from build123d import *

# Parameters (mm, degrees)
ESBO_O1_R                = 40
RESSALTO_EXTRUS_O1_DEPTH = 1
ESBO_O3_R                = 3.5
RESSALTO_EXTRUS_O2_DEPTH = 2
ESBO_O4_R                = 2.5
CORTE_EXTRUS_O2_DEPTH    = 2
CHANFRO1_SIZE            = 2
ESBO_O6_R                = 1.1
CORTE_EXTRUS_O4_DEPTH    = 3
CORTE_EXTRUS_O5_START    = -3
CORTE_EXTRUS_O5_DEPTH    = 3
ESBO_O7_W                = 38.307647293
ESBO_O7_H                = 77.740133008
CORTE_EXTRUS_O6_DEPTH    = 3
FILETE1_R                = 20
FILETE2_R                = 20


with BuildPart() as part:
    # Esboço1 → Ressalto-extrusão1 (new body)
    with BuildSketch(Plane(origin=(0, 0, 0), x_dir=(1, 0, 0), z_dir=(0, 1, 0))):
        with Locations(Location((0, 0, 0), (0, 0, 270))):
            Circle(ESBO_O1_R)
    extrude(amount=RESSALTO_EXTRUS_O1_DEPTH)

    # Esboço3 → Ressalto-extrusão2 (add)
    with BuildSketch(Plane(origin=(0, 1, 0), x_dir=(1, 0, 0), z_dir=(0, 1, 0))):
        with Locations(Location((0, 0, 0), (0, 0, 270))):
            Circle(ESBO_O3_R)
    extrude(amount=RESSALTO_EXTRUS_O2_DEPTH)

    # Esboço4 → Corte-extrusão2 (cut)
    with BuildSketch(Plane(origin=(0, 3, 0), x_dir=(1, 0, 0), z_dir=(0, 1, 0))):
        with Locations(Location((0, 0, 0), (0, 0, 270))):
            Circle(ESBO_O4_R)
    extrude(amount=-CORTE_EXTRUS_O2_DEPTH, mode=Mode.SUBTRACT)

    # Chanfro1
    chanfro1_edges = [part.edges().sort_by_distance(p)[0] for p in [
        (0, 1, -3.5),
    ]]
    chamfer(chanfro1_edges, length=CHANFRO1_SIZE - 0.0001)  # a hair under: the kernel refuses the full size

    # Esboço6 → Corte-extrusão4 (cut)
    with BuildSketch(Plane(origin=(0, 1, 0), x_dir=(1, 0, 0), z_dir=(0, 1, 0))):
        with Locations(Location((0, 0, 0), (0, 0, 270))):
            Circle(ESBO_O6_R)
    extrude(amount=-CORTE_EXTRUS_O4_DEPTH, mode=Mode.SUBTRACT)

    # Esboço2 → Corte-extrusão5 (cut)
    with BuildSketch(Plane(origin=(0, 1, 0), x_dir=(1, 0, 0), z_dir=(0, 1, 0)).offset(CORTE_EXTRUS_O5_START)):
        with BuildLine():
            ThreePointArc((20, 4), (16, 0), (20, -4))
            Line((20, -4), (39.223227028, -7.844645406))
            ThreePointArc((39.223227028, -7.844645406), (40, 0), (39.223227028, 7.844645406))
            Line((39.223227028, 7.844645406), (20, 4))
        make_face()
    extrude(amount=CORTE_EXTRUS_O5_DEPTH, mode=Mode.SUBTRACT)

    # Esboço7 → Corte-extrusão6 (cut)
    with BuildSketch(Plane(origin=(0, 1, 0), x_dir=(1, 0, 0), z_dir=(0, 1, 0))):
        with Locations((-28.594052983, 0)):
            Rectangle(ESBO_O7_W, ESBO_O7_H)
    extrude(amount=-CORTE_EXTRUS_O6_DEPTH, mode=Mode.SUBTRACT)

    # Filete1
    filete1_edges = [part.edges().sort_by_distance(p)[0] for p in [
        (-9.440229337, 0.5, -38.870066504),
    ]]
    fillet(filete1_edges, radius=FILETE1_R)

    # Filete2
    filete2_edges = [part.edges().sort_by_distance(p)[0] for p in [
        (-9.440229337, 0.5, 38.870066504),
    ]]
    fillet(filete2_edges, radius=FILETE2_R)


solid = part.part
Design review of the part built by this model. Coordinates are the model's own, in mm. A direction names the side the tool comes from. Coordinates: 2 decimals unless noted, no trailing zeros. Write each loop counter-clockwise with the first axis right and the second up, starting at its lowest first coordinate (ties: lowest second). Pieces come first, ordered by that corner, then holes. Notation, with made-up numbers: (39.5, -27) - (67.5, -27) arc R19 ccw to (67.5, -22) - close; hole circle Ø11 at (68.25, 27). An arc over 180 degrees is marked (long way). One line per item, written item: value.
1) For faces 1 (the face through (-2.44, 2.01, -0.54)), 2 (the face through (29.75, 0.49, -5.95)), 3 (the face through (1.09, 0.51, -0.14)), list the 3-axis set-ups (+Z, -Z, +X, -X, +Y, -Y) from which the entire face can be reached by the end or side of a thin tool; tool diameter is ignored.
Answer sheet:
face 1: +Y
face 2: +X, +Y, -Y
face 3: +Y, -Y
2) Add section D-D (z = -16). State the section outline as (x, y) points, plus the area to 3 significant figures.
Answer sheet:
outline: (-9.44, 0) - (36.66, 0) - (36.66, 1) - (-9.44, 1) - close
area: 46.1 mm2
3) Add section A-A (x = 24). State the section outline as (y, z) points.
Answer sheet:
outline: (0, -32) - (1, -32) - (1, -4.8) - (0, -4.8) - close; (0, 4.8) - (1, 4.8) - (1, 32) - (0, 32) - close
4) Insertion check: pin 1 (8 mm diameter, centred on x = 25.5, z = -3.5, fed in from -Y); pin 2 (1 mm diameter, centred on x = 11, z = 29, fed in from +Y); pin 3 (1.5 mm diameter, centred on x = 6, y = 1, fed in from +Z). Each pin has a flat end and moves straight along its axis. Give the tip position at first contact, or say it passes through.
Answer sheet:
pin 1: stops at y = 0
pin 2: stops at y = 1
pin 3: stops at z = 36.62
5) Mouldability with a two-part tool opening along X and no side actions: class faces 4 (the face through (-1, 1, 1)), 5 (the face through (33.01, 0.49, -22.59)), 6 (the face through (10, 1, -1)) as +X half, -X half, draft (parallel to the pull), parting line (faces both ways), or undercut.
Answer sheet:
face 4: undercut
face 5: +X half
face 6: draft
6) To check wall thickness, follow probe 1 along X at (y, z) = (0.55, 0); probe 2 along Y at (x, z) = (14, 5.5); probe 3 along X at (y, z) = (2.5, 0). State the ranges of each line that lie inside material, in increasing order.
Answer sheet:
probe 1: x = -9.44 to -1.1, 1.1 to 16
probe 2: y = 0 to 1
probe 3: x = -4 to -2.5, 2.5 to 4
7) Add section C-C (y = 1.65). State the section outline as (x, z) points, plus the area to 3 significant figures.
Answer sheet:
outline: circle Ø9.7 at (0, 0); hole circle Ø5 at (0, 0)
area: 54.3 mm2
